Source: three-view drawing plus pictorial views. Frame: mm from the lowest corner of the part. Round coordinates to 2 decimals unless told otherwise and drop trailing zeros. Write each loop counter-clockwise with the first axis right and the second up, starting at its lowest first coordinate (ties: lowest second). Pieces come first, ordered by that corner, then holes.
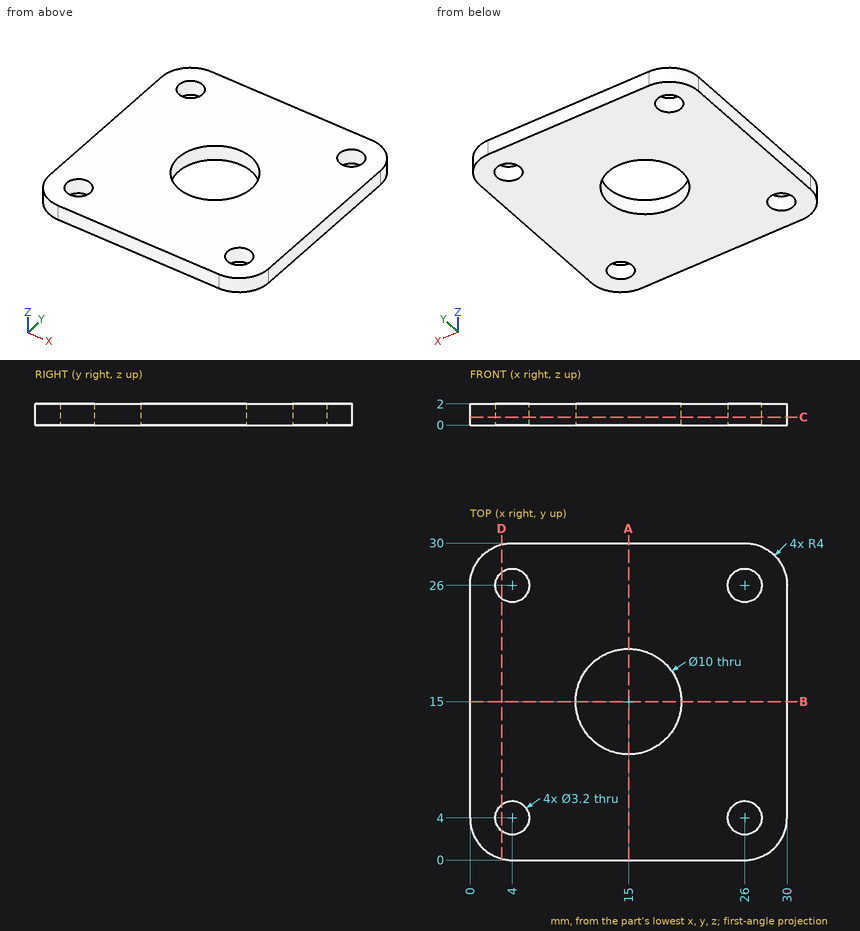
1) Section A-A on x = 15. Output: boundary loops of the cut face in (y, z), plus the area to 3 significant figures.
2) Section D-D on x = 3. Output: boundary loops of the cut face in (y, z).
3) First-contact query: P1, Ø4, axis at x = 25.5, y = 7.5, coming from the -Z side; P2, Ø3, axis at x = 26, y = 4, coming from the -Z side. Flat tips, straight axial feed; report the tip coordinate or a pass-through.
4) Section C-C on z = 0.75. Output: boundary loops of the cut face in (x, y).
5) Line query: probe 1 along X at (y, z) = (26, 0.95); probe 2 along Y at (x, z) = (14.75, 1.05). Output: solid intervals per line, ascending.
Filled in:
1. outline: (0, 0) - (10, 0) - (10, 2) - (0, 2) - close; (20, 0) - (30, 0) - (30, 2) - (20, 2) - close
1. area: 40.0 mm2
2. outline: (0.13, 0) - (2.75, 0) - (2.75, 2) - (0.13, 2) - close; (5.25, 0) - (24.75, 0) - (24.75, 2) - (5.25, 2) - close; (27.25, 0) - (29.87, 0) - (29.87, 2) - (27.25, 2) - close
3. P1: stops at z = 0
3. P2: passes through
4. outline: (0, 4) arc R4 ccw to (4, 0) - (26, 0) arc R4 ccw to (30, 4) - (30, 26) arc R4 ccw to (26, 30) - (4, 30) arc R4 ccw to (0, 26) - close; hole circle Ø3.2 at (4, 4); hole circle Ø3.2 at (4, 26); hole circle Ø10 at (15, 15); hole circle Ø3.2 at (26, 4); hole circle Ø3.2 at (26, 26)
5. probe 1: x = 0 to 2.4, 5.6 to 24.4, 27.6 to 30
5. probe 2: y = 0 to 10.01, 19.99 to 30
